The listing builds one solid part. Answer for the finished solid, in the listing's coordinates (mm). Face numbers are marked on the shaded views. A direction names the side the tool comes from. Round coordinates to 2 decimals unless told otherwise and drop trailing zeros. Write each loop counter-clockwise with the first axis right and the second up, starting at its lowest first coordinate (ties: lowest second). Pieces come first, ordered by that corner, then holes. Notation, with made-up numbers: M -14.5,-11 L 2.5,-11 A23 ccw 2.5,25 Z; hole C 15,24.5 d4. An arc over 180 degrees is marked long. One line per item, written item: value. Start each with the question number.
(1) Consider probe 1 along X at (y, z) = (-10, 10.6); probe 2 along Y at (x, z) = (9.5, 6.25); probe 3 along Z at (x, y) = (21.25, -10). Determine where each line is inside the solid, lowest interval first.
(2) Given P1, Ø4, axis at x = 5.5, y = -10, coming from the -Z side; P2, Ø3, axis at x = 16.5, y = -10, coming from the +Z side; P3, Ø2, axis at x = 5.5, y = -10, coming from the +Z side, each flat-ended and moving along its own axis, determine where each tip first touches the part or whether it passes through.
(3) Section A-A (x = 27) is taken. Determine the outline of the cut face in (y, z).
(4) For the marked faces 4 and 5, determine the directions among +Z, -Z, +X, -X, +Y, -Y from which every point of the face is accessible in a straight line to the end or side of a thin tool.
(5) Section B-B (z = 6) is taken. Determine the outline of the cut face in (x, y), plus the area to 3 significant figures.
(6) Section D-D (y = -10) is taken. State how many separate pieces and enclosed holes the cut face has, plus the area to 3 significant figures.
(7) Section C-C (y = -17) is taken. Determine the outline of the cut face in (x, z), plus the area to 3 significant figures.
(8) For a pull along Z with two mould halves and no side action, classify the marked faces 1, 2 and 3 as released by +Z, released by -Z, zero draft, split by the parting line, or undercut.
```python
from build123d import *

# Parameters (mm, degrees)
F0_W      = 30
F0_H      = 20
F1_DEPTH  = 12
F2_R      = 4
F3_DEPTH  = 30
F4_R      = 1.25
F5_DEPTH  = 25
F4_R_2    = 1.05
F8_DEPTH  = 25
F9_SIZE   = 0.25
F4_R_3    = 3.5
F4_R_4    = 2.5
F10_DEPTH = 0.6


with BuildPart() as f1:
    # F0 (on Top) → F1 (new body)
    with BuildSketch(Plane.XY):
        with Locations((15, -10)):
            Rectangle(F0_W, F0_H)
    extrude(amount=F1_DEPTH)

    # F2 (on face) → F3 (cut)
    with BuildSketch(Plane(origin=(0, 0, 0), x_dir=(0, -1, 0), z_dir=(-1, 0, 0))):
        with Locations((10, 6)):
            Circle(F2_R)
    extrude(amount=-F3_DEPTH, mode=Mode.SUBTRACT)

    # F4 (on face) → F5 (cut)
    with BuildSketch(Plane.XY.offset(12)):
        with Locations((5.5, -10)):
            Circle(F4_R)
        with Locations((16.5, -10)):
            Circle(F4_R)
    extrude(amount=-F5_DEPTH, mode=Mode.SUBTRACT)

    # F4 (on face) → F8 (cut)
    with BuildSketch(Plane.XY.offset(12)):
        with Locations((3, -17)):
            Circle(F4_R_2)
        with Locations((27, -3)):
            Circle(F4_R_2)
    extrude(amount=-F8_DEPTH, mode=Mode.SUBTRACT)

    # F9
    f9_edges = [f1.edges().sort_by_distance(p)[0] for p in [
        (0, -6, 6),
        (0, 0, 6),
        (0, -20, 6),
        (30, 0, 6),
        (30, -20, 6),
    ]]
    chamfer(f9_edges, length=F9_SIZE)

    # F4 (on face) → F10 (cut)
    with BuildSketch(Plane.XY.offset(12)):
        with Locations((5.5, -10)):
            Circle(F4_R_3)
        with Locations((5.5, -10)):
            Circle(F4_R_4, mode=Mode.SUBTRACT)
        with Locations((16.5, -10)):
            Circle(F4_R_3)
        with Locations((16.5, -10)):
            Circle(F4_R_4, mode=Mode.SUBTRACT)
        with Locations((16.5, -10)):
            Circle(F4_R_4)
        with Locations((16.5, -10)):
            Circle(F4_R, mode=Mode.SUBTRACT)
        with Locations((5.5, -10)):
            Circle(F4_R_4)
        with Locations((5.5, -10)):
            Circle(F4_R, mode=Mode.SUBTRACT)
    extrude(amount=-F10_DEPTH, mode=Mode.SUBTRACT)


solid = f1.part
```
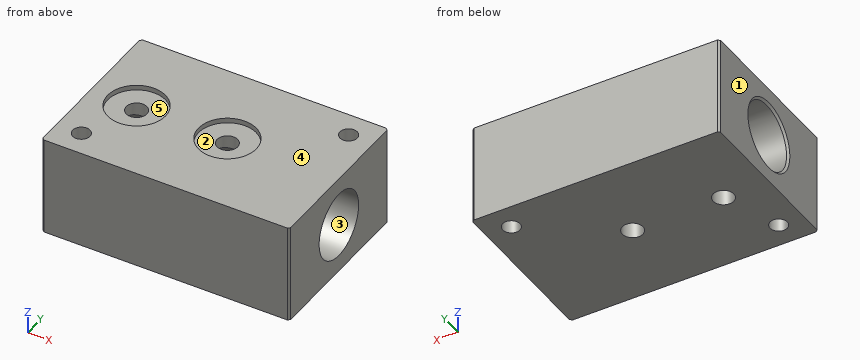
Recorded:
1. probe 1: x = 0 to 4.25, 6.75 to 15.25, 17.75 to 30
1. probe 2: y = -20 to -13.99, -6.01 to 0
1. probe 3: z = 0 to 2, 10 to 12
2. P1: stops at z = 0
2. P2: stops at z = 11.4
2. P3: passes through
3. outline: M -20,0 L -4.05,0 L -4.05,12 L -20,12 Z; M -1.95,0 L 0,0 L 0,12 L -1.95,12 Z; hole C -10,6 d8
4. face 4: +Z, +X, -X, +Y, -Y
4. face 5: +Z
5. outline: M 0,-19.75 L 0.25,-20 L 29.75,-20 L 30,-19.75 L 30,-14 L 0.25,-14 L 0,-14.25 Z; M 0,-5.75 L 0.25,-6 L 30,-6 L 30,-0.25 L 29.75,0 L 0.25,0 L 0,-0.25 Z; hole C 3,-17 d2.1; hole C 27,-3 d2.1
5. area: 353 mm2
6. separate pieces: 6
6. enclosed holes: 0
6. area: 94.5 mm2
7. outline: M 0,0 L 1.95,0 L 1.95,12 L 0,12 Z; M 4.05,0 L 30,0 L 30,12 L 4.05,12 Z
7. area: 335 mm2
8. face 1: zero draft
8. face 2: released by +Z
8. face 3: undercut
